The model under review builds one solid part; all positions refer to its coordinate system, in mm. A direction names the side the tool comes from. Give positions to 0.01 mm unless a question says otherwise; leave off trailing zeros. Write each loop counter-clockwise with the first axis right and the second up, starting at its lowest first coordinate (ties: lowest second). Pieces come first, ordered by that corner, then holes. Notation, with made-up numbers: M 81,62.5 L 88,62.5 A17 cw 88,85.5 Z; hole C -31,-33.75 d11. An arc over 180 degrees is marked long. Write item = value, one per line. Start each with the question number.
Autodesk Inventor part; units mm, degrees
ref_plane "YZ Plane" through (0, 0, 0) normal (1, 0, 0) x (0, 1, 0)
ref_plane "XZ Plane" through (0, 0, 0) normal (0, 1, 0) x (-1, 0, 0)
ref_plane "XY Plane" through (0, 0, 0) normal (0, 0, 1) x (1, 0, 0)
sketch "草圖1" plane through (0, 0, 0) normal (0, 0, 1) x (1, 0, 0)
  line L0 (0, 0) -> (20, 0)
  line L1 (20, 0) -> (20, -36.5)
  line L2 (20, -36.5) -> (0, -36.5)
  line L3 (0, -36.5) -> (0, 0)
  dimension "d0" = 20
  dimension "d1" = 36.5
extrude "擠出1" add sketch "草圖1" along normal blind 2
sketch "草圖2" plane through (0, 0, 2) normal (0, 0, 1) x (1, 0, 0)
  line L0 (1, -1) -> (19, -1)
  line L1 (19, -1) -> (19, -35.5)
  line L2 (19, -35.5) -> (1, -35.5)
  line L3 (1, -35.5) -> (1, -1)
  line L4 (20, 0) -> (0, 0)
  line L5 (20, -36.5) -> (20, 0)
  line L6 (0, -36.5) -> (20, -36.5)
  line L7 (0, 0) -> (0, -36.5)
  dimension "d4" = 1
  dimension "d5" = 1
  dimension "d6" = 1
  dimension "d7" = 1
extrude "擠出2" add sketch "草圖2" along normal blind 2 contours L0 L1 L2 L3
sketch "草圖3" plane through (0, 0, 4) normal (0, 0, 1) x (1, 0, 0)
  line L0 (20, -36.5) -> (20, 0)
  line L1 (0, 0) -> (20, 0)
  line L2 (20, 0) -> (20, -36.5)
  line L3 (20, -36.5) -> (0, -36.5)
  line L4 (0, -36.5) -> (0, 0)
extrude "擠出3" add sketch "草圖3" along normal blind 2
sketch "草圖4" plane through (0, 0, 6) normal (0, 0, 1) x (1, 0, 0)
  line L0 (1, -35.5) -> (1, -1)
  line L1 (19, -1) -> (19, -35.5)
  line L2 (1, -1) -> (19, -1)
  line L3 (19, -1) -> (19, -35.5)
  line L4 (19, -35.5) -> (1, -35.5)
  line L5 (1, -35.5) -> (1, -1)
  point P0 (0, 0)
extrude "擠出4" add sketch "草圖4" along normal blind 2
sketch "草圖5" plane through (0, 0, 8) normal (0, 0, 1) x (1, 0, 0)
  line L0 (20, -36.5) -> (20, 0)
  line L1 (0, 0) -> (20, 0)
  line L2 (20, 0) -> (20, -36.5)
  line L3 (20, -36.5) -> (0, -36.5)
  line L4 (0, -36.5) -> (0, 0)
extrude "擠出5" add sketch "草圖5" along normal blind 2
sketch "草圖6" plane through (0, 0, 10) normal (0, 0, 1) x (1, 0, 0)
  line L0 (1, -1) -> (19, -1)
  line L1 (19, -35.5) -> (1, -35.5)
  line L2 (1, -1) -> (19, -1)
  line L3 (19, -1) -> (19, -35.5)
  line L4 (19, -35.5) -> (1, -35.5)
  line L5 (1, -35.5) -> (1, -1)
  point P0 (0, 0)
extrude "擠出6" add sketch "草圖6" along normal blind 2
sketch "草圖7" plane through (0, 0, 0) normal (0, 0, -1) x (-1, 0, 0)
  line L0 (-19, -1) -> (-19, -35.5)
  line L1 (-1, -1) -> (-1, -35.5)
  line L2 (-19, -1) -> (-1, -1)
  line L3 (-1, -1) -> (-1, -35.5)
  line L4 (-1, -35.5) -> (-19, -35.5)
  line L5 (-19, -35.5) -> (-19, -1)
  point P0 (0, 0)
extrude "擠出7" add sketch "草圖7" along normal blind 2
sketch "草圖8" plane through (0, 0, -2) normal (0, 0, -1) x (-1, 0, 0)
  line L0 (0, 0) -> (0, -36.5)
  line L1 (-20, 0) -> (0, 0)
  line L2 (0, 0) -> (0, -36.5)
  line L3 (0, -36.5) -> (-20, -36.5)
  line L4 (-20, -36.5) -> (-20, 0)
extrude "擠出8" add sketch "草圖8" along normal blind 2
sketch "草圖9" plane through (0, 0, -4) normal (0, 0, -1) x (-1, 0, 0)
  line L0 (-1, -1) -> (-1, -35.5)
  line L1 (-19, -1) -> (-1, -1)
  line L2 (-1, -1) -> (-1, -35.5)
  line L3 (-1, -35.5) -> (-19, -35.5)
  line L4 (-19, -35.5) -> (-19, -1)
  point P0 (0, 0)
extrude "擠出9" add sketch "草圖9" along normal blind 2
sketch "草圖10" plane through (0, 0, -6) normal (0, 0, -1) x (-1, 0, 0)
  line L0 (0, 0) -> (-20, 0)
  line L1 (0, -36.5) -> (0, 0)
  line L2 (-20, 0) -> (0, 0)
  line L3 (0, 0) -> (0, -36.5)
  line L4 (0, -36.5) -> (-20, -36.5)
  line L5 (-20, -36.5) -> (-20, 0)
extrude "擠出10" add sketch "草圖10" along normal blind 2
properties part number "連接件1"
Item 1: We need section A-A, the plane z = -5.5. Write out the cut boundary in (x, y).
Item 2: For faces 5 (the flat face through (1, -18, 11)), 6 (the flat face through (10, -1, 11)), 7 (the flat face through (1, -18, 7)), 8 (the flat face through (10, -1, 3)), 9 (the flat face through (10, -35.5, 11)), list the 3-axis set-ups (+Z, -Z, +X, -X, +Y, -Y) from which the entire face can be reached by the end or side of a thin tool; tool diameter is ignored.
Item 3: The part is to be moulded in two halves that separate along Z. For faces 1 (the flat face through (0, -19, 5)), 2 (the flat face through (19.7, -18.2, -6)), 3 (the flat face through (10, -18, 12)), 4 (the flat face through (0.3, -18.2, 6)), say which applies: released by +Z, released by -Z, zero draft, split by the parting line, or undercut.
Item 4: Clearance check with flat-ended pins moving along their axes: P1, Ø0.6, axis at y = -22, z = 11, coming from the +X side; P2, Ø1.6, axis at x = 13, z = 11, coming from the -Y side; P3, Ø1, axis at y = -10.5, z = 11, coming from the -X side. State where each tip first meets the part, or that it passes through.
Item 5: To check wall thickness, follow probe 1 along Y at (x, z) = (2, -4.5); probe 2 along X at (y, z) = (-30, -5.75). State the ranges of each line that lie inside material, in increasing order. Write a range as [from, to].
Worked out:
q1.outline = M 1,-35.5 L 19,-35.5 L 19,-1 L 1,-1 Z
q2.face_5 = +Z, -X, +Y, -Y
q2.face_6 = +Z, +X, -X, +Y
q2.face_7 = -X, +Y, -Y
q2.face_8 = +X, -X, +Y
q2.face_9 = +Z, +X, -X, -Y
q3.face_1 = zero draft
q3.face_2 = undercut
q3.face_3 = released by +Z
q3.face_4 = undercut
q4.P1 = 19
q4.P2 = -35.5
q4.P3 = 1
q5.probe_1 = [-35.5, -1]
q5.probe_2 = [1, 19]
